Geometry: final body of the model. Coordinates: model frame, mm. Give positions to 0.01 mm unless a question says otherwise; leave off trailing zeros. Write each loop counter-clockwise with the first axis right and the second up, starting at its lowest first coordinate (ties: lowest second). Pieces come first, ordered by that corner, then holes. Notation, with made-up numbers: M 8,55 L 55,55 A23 cw 55,81 Z; hole C -18,51.5 d6. An arc over 180 degrees is marked long. Answer as a JSON object with one key per item and string values.
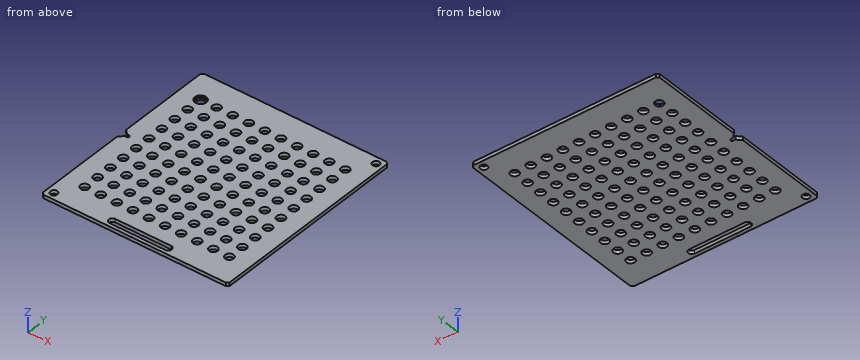
from build123d import *

# Parameters (mm, degrees)
F0_R     = 5
F0_R_2   = 6
F0_R_3   = 8.1
F1_DEPTH = 5
F2_DEPTH = 3


with BuildPart() as f1:
    # F0 (on Top) → F1 (new body)
    with BuildSketch(Plane.XY):
        with BuildLine():
            Line((133.5, 140.5), (130.5, 143.5))
            Line((130.5, 143.5), (-130.5, 143.5))
            Line((-130.5, 143.5), (-133.5, 140.5))
            Line((-133.5, 140.5), (-133.5, 8))
            Line((-133.5, 8), (-127.5, 2))
            Line((-127.5, 2), (-124.5, 2))
            ThreePointArc((-124.5, 2), (-122.5, 0), (-124.5, -2))
            Line((-124.5, -2), (-127.5, -2))
            Line((-127.5, -2), (-133.5, -8))
            Line((-133.5, -8), (-133.5, -140.5))
            Line((-133.5, -140.5), (-130.5, -143.5))
            Line((-130.5, -143.5), (130.5, -143.5))
            Line((130.5, -143.5), (133.5, -140.5))
            Line((133.5, -140.5), (133.5, 140.5))
        make_face()
        with Locations((-123.5, -133.5)):
            Circle(F0_R, mode=Mode.SUBTRACT)
        with Locations((-103.5, -103.5)):
            Circle(F0_R_2, mode=Mode.SUBTRACT)
        with Locations((-103.5, -80.5)):
            Circle(F0_R_2, mode=Mode.SUBTRACT)
        with Locations((-80.5, -103.5)):
            Circle(F0_R_2, mode=Mode.SUBTRACT)
        with Locations((-80.5, -80.5)):
            Circle(F0_R_2, mode=Mode.SUBTRACT)
        with Locations((-57.5, -103.5)):
            Circle(F0_R_2, mode=Mode.SUBTRACT)
        with Locations((-34.5, -103.5)):
            Circle(F0_R_2, mode=Mode.SUBTRACT)
        with Locations((-57.5, -80.5)):
            Circle(F0_R_2, mode=Mode.SUBTRACT)
        with Locations((-34.5, -80.5)):
            Circle(F0_R_2, mode=Mode.SUBTRACT)
        with Locations((-11.5, -103.5)):
            Circle(F0_R_2, mode=Mode.SUBTRACT)
        with Locations((-11.5, -80.5)):
            Circle(F0_R_2, mode=Mode.SUBTRACT)
        with Locations((-103.5, -57.5)):
            Circle(F0_R_2, mode=Mode.SUBTRACT)
        with Locations((-80.5, -57.5)):
            Circle(F0_R_2, mode=Mode.SUBTRACT)
        with Locations((-103.5, -34.5)):
            Circle(F0_R_2, mode=Mode.SUBTRACT)
        with Locations((-103.5, -11.5)):
            Circle(F0_R_2, mode=Mode.SUBTRACT)
        with Locations((-80.5, -34.5)):
            Circle(F0_R_2, mode=Mode.SUBTRACT)
        with Locations((-80.5, -11.5)):
            Circle(F0_R_2, mode=Mode.SUBTRACT)
        with Locations((-57.5, -57.5)):
            Circle(F0_R_2, mode=Mode.SUBTRACT)
        with Locations((-34.5, -57.5)):
            Circle(F0_R_2, mode=Mode.SUBTRACT)
        with Locations((-11.5, -57.5)):
            Circle(F0_R_2, mode=Mode.SUBTRACT)
        with Locations((-57.5, -34.5)):
            Circle(F0_R_2, mode=Mode.SUBTRACT)
        with Locations((-34.5, -34.5)):
            Circle(F0_R_2, mode=Mode.SUBTRACT)
        with Locations((-57.5, -11.5)):
            Circle(F0_R_2, mode=Mode.SUBTRACT)
        with Locations((-34.5, -11.5)):
            Circle(F0_R_2, mode=Mode.SUBTRACT)
        with Locations((-11.5, -34.5)):
            Circle(F0_R_2, mode=Mode.SUBTRACT)
        with Locations((-11.5, -11.5)):
            Circle(F0_R_2, mode=Mode.SUBTRACT)
        with BuildLine():
            Line((40, -138.5), (-40, -138.5))
            ThreePointArc((-40, -138.5), (-45, -133.5), (-40, -128.5))
            Line((-40, -128.5), (40, -128.5))
            ThreePointArc((40, -128.5), (45, -133.5), (40, -138.5))
        make_face(mode=Mode.SUBTRACT)
        with Locations((11.5, -103.5)):
            Circle(F0_R_2, mode=Mode.SUBTRACT)
        with Locations((11.5, -80.5)):
            Circle(F0_R_2, mode=Mode.SUBTRACT)
        with Locations((34.5, -103.5)):
            Circle(F0_R_2, mode=Mode.SUBTRACT)
        with Locations((57.5, -103.5)):
            Circle(F0_R_2, mode=Mode.SUBTRACT)
        with Locations((34.5, -80.5)):
            Circle(F0_R_2, mode=Mode.SUBTRACT)
        with Locations((57.5, -80.5)):
            Circle(F0_R_2, mode=Mode.SUBTRACT)
        with Locations((80.5, -103.5)):
            Circle(F0_R_2, mode=Mode.SUBTRACT)
        with Locations((80.5, -80.5)):
            Circle(F0_R_2, mode=Mode.SUBTRACT)
        with Locations((103.5, -103.5)):
            Circle(F0_R_2, mode=Mode.SUBTRACT)
        with Locations((103.5, -80.5)):
            Circle(F0_R_2, mode=Mode.SUBTRACT)
        with Locations((11.5, -57.5)):
            Circle(F0_R_2, mode=Mode.SUBTRACT)
        with Locations((34.5, -57.5)):
            Circle(F0_R_2, mode=Mode.SUBTRACT)
        with Locations((57.5, -57.5)):
            Circle(F0_R_2, mode=Mode.SUBTRACT)
        with Locations((11.5, -34.5)):
            Circle(F0_R_2, mode=Mode.SUBTRACT)
        with Locations((11.5, -11.5)):
            Circle(F0_R_2, mode=Mode.SUBTRACT)
        with Locations((34.5, -34.5)):
            Circle(F0_R_2, mode=Mode.SUBTRACT)
        with Locations((57.5, -34.5)):
            Circle(F0_R_2, mode=Mode.SUBTRACT)
        with Locations((34.5, -11.5)):
            Circle(F0_R_2, mode=Mode.SUBTRACT)
        with Locations((57.5, -11.5)):
            Circle(F0_R_2, mode=Mode.SUBTRACT)
        with Locations((80.5, -57.5)):
            Circle(F0_R_2, mode=Mode.SUBTRACT)
        with Locations((103.5, -57.5)):
            Circle(F0_R_2, mode=Mode.SUBTRACT)
        with Locations((80.5, -34.5)):
            Circle(F0_R_2, mode=Mode.SUBTRACT)
        with Locations((80.5, -11.5)):
            Circle(F0_R_2, mode=Mode.SUBTRACT)
        with Locations((103.5, -34.5)):
            Circle(F0_R_2, mode=Mode.SUBTRACT)
        with Locations((103.5, -11.5)):
            Circle(F0_R_2, mode=Mode.SUBTRACT)
        with Locations((-103.5, 11.5)):
            Circle(F0_R_2, mode=Mode.SUBTRACT)
        with Locations((-103.5, 34.5)):
            Circle(F0_R_2, mode=Mode.SUBTRACT)
        with Locations((-80.5, 11.5)):
            Circle(F0_R_2, mode=Mode.SUBTRACT)
        with Locations((-80.5, 34.5)):
            Circle(F0_R_2, mode=Mode.SUBTRACT)
        with Locations((-103.5, 57.5)):
            Circle(F0_R_2, mode=Mode.SUBTRACT)
        with Locations((-80.5, 57.5)):
            Circle(F0_R_2, mode=Mode.SUBTRACT)
        with Locations((-57.5, 11.5)):
            Circle(F0_R_2, mode=Mode.SUBTRACT)
        with Locations((-34.5, 11.5)):
            Circle(F0_R_2, mode=Mode.SUBTRACT)
        with Locations((-57.5, 34.5)):
            Circle(F0_R_2, mode=Mode.SUBTRACT)
        with Locations((-34.5, 34.5)):
            Circle(F0_R_2, mode=Mode.SUBTRACT)
        with Locations((-11.5, 11.5)):
            Circle(F0_R_2, mode=Mode.SUBTRACT)
        with Locations((-11.5, 34.5)):
            Circle(F0_R_2, mode=Mode.SUBTRACT)
        with Locations((-57.5, 57.5)):
            Circle(F0_R_2, mode=Mode.SUBTRACT)
        with Locations((-34.5, 57.5)):
            Circle(F0_R_2, mode=Mode.SUBTRACT)
        with Locations((-11.5, 57.5)):
            Circle(F0_R_2, mode=Mode.SUBTRACT)
        with Locations((-103.5, 80.5)):
            Circle(F0_R_2, mode=Mode.SUBTRACT)
        with Locations((-103.5, 103.5)):
            Circle(F0_R_3, mode=Mode.SUBTRACT)
        with Locations((-80.5, 80.5)):
            Circle(F0_R_2, mode=Mode.SUBTRACT)
        with Locations((-80.5, 103.5)):
            Circle(F0_R_2, mode=Mode.SUBTRACT)
        with Locations((-57.5, 80.5)):
            Circle(F0_R_2, mode=Mode.SUBTRACT)
        with Locations((-34.5, 80.5)):
            Circle(F0_R_2, mode=Mode.SUBTRACT)
        with Locations((-57.5, 103.5)):
            Circle(F0_R_2, mode=Mode.SUBTRACT)
        with Locations((-34.5, 103.5)):
            Circle(F0_R_2, mode=Mode.SUBTRACT)
        with Locations((-11.5, 80.5)):
            Circle(F0_R_2, mode=Mode.SUBTRACT)
        with Locations((-11.5, 103.5)):
            Circle(F0_R_2, mode=Mode.SUBTRACT)
        with Locations((11.5, 11.5)):
            Circle(F0_R_2, mode=Mode.SUBTRACT)
        with Locations((11.5, 34.5)):
            Circle(F0_R_2, mode=Mode.SUBTRACT)
        with Locations((34.5, 11.5)):
            Circle(F0_R_2, mode=Mode.SUBTRACT)
        with Locations((57.5, 11.5)):
            Circle(F0_R_2, mode=Mode.SUBTRACT)
        with Locations((34.5, 34.5)):
            Circle(F0_R_2, mode=Mode.SUBTRACT)
        with Locations((57.5, 34.5)):
            Circle(F0_R_2, mode=Mode.SUBTRACT)
        with Locations((11.5, 57.5)):
            Circle(F0_R_2, mode=Mode.SUBTRACT)
        with Locations((34.5, 57.5)):
            Circle(F0_R_2, mode=Mode.SUBTRACT)
        with Locations((57.5, 57.5)):
            Circle(F0_R_2, mode=Mode.SUBTRACT)
        with Locations((80.5, 11.5)):
            Circle(F0_R_2, mode=Mode.SUBTRACT)
        with Locations((80.5, 34.5)):
            Circle(F0_R_2, mode=Mode.SUBTRACT)
        with Locations((103.5, 11.5)):
            Circle(F0_R_2, mode=Mode.SUBTRACT)
        with Locations((103.5, 34.5)):
            Circle(F0_R_2, mode=Mode.SUBTRACT)
        with Locations((80.5, 57.5)):
            Circle(F0_R_2, mode=Mode.SUBTRACT)
        with Locations((103.5, 57.5)):
            Circle(F0_R_2, mode=Mode.SUBTRACT)
        with Locations((11.5, 80.5)):
            Circle(F0_R_2, mode=Mode.SUBTRACT)
        with Locations((11.5, 103.5)):
            Circle(F0_R_2, mode=Mode.SUBTRACT)
        with Locations((34.5, 80.5)):
            Circle(F0_R_2, mode=Mode.SUBTRACT)
        with Locations((57.5, 80.5)):
            Circle(F0_R_2, mode=Mode.SUBTRACT)
        with Locations((34.5, 103.5)):
            Circle(F0_R_2, mode=Mode.SUBTRACT)
        with Locations((57.5, 103.5)):
            Circle(F0_R_2, mode=Mode.SUBTRACT)
        with Locations((80.5, 80.5)):
            Circle(F0_R_2, mode=Mode.SUBTRACT)
        with Locations((80.5, 103.5)):
            Circle(F0_R_2, mode=Mode.SUBTRACT)
        with Locations((103.5, 80.5)):
            Circle(F0_R_2, mode=Mode.SUBTRACT)
        with Locations((103.5, 103.5)):
            Circle(F0_R_2, mode=Mode.SUBTRACT)
        with Locations((123.5, 133.5)):
            Circle(F0_R, mode=Mode.SUBTRACT)
    extrude(amount=F1_DEPTH)

    # F0 (on Top) → F2 (join)
    with BuildSketch(Plane.XY):
        with Locations((-103.5, 103.5)):
            Circle(F0_R_3)
        with Locations((-103.5, 103.5)):
            Circle(F0_R_2, mode=Mode.SUBTRACT)
    extrude(amount=F2_DEPTH)


solid = f1.part
1) Contact query for flat-ended pins moving along their axis: P1, Ø19, axis at x = 34.5, y = 80.5, coming from the -Z side; P2, Ø9.5, axis at x = 11.5, y = 103.5, coming from the -Z side. Output: stop coordinate, or through.
Geometry check:
{"P1": "stops at z = 0", "P2": "passes through"}
2) Cut plane A-A on x = -21. Return loops of the section in (y, z), and give its area (4 significant figures).
Geometry check:
{"outline": "M -143.5,0 L -138.5,0 L -138.5,5 L -143.5,5 Z; M -128.5,0 L 143.5,0 L 143.5,5 L -128.5,5 Z", "area": "1,385 mm2"}
3) Cut plane B-B on y = 11.5. Give the number of separate pieces and of enclosed holes in the cut face, and give its area (3 significant figures).
Geometry check:
{"separate pieces": "11", "enclosed holes": "0", "area": "735 mm2"}
